Input: part model. Units: mm. Frame: model coordinates. Coordinates: 2 decimals unless noted, no trailing zeros. Loops run counter-clockwise (first coordinate to the right, second up) from the corner with the lowest first, then second, coordinate; pieces in that order, holes last.
```python
from build123d import *

# Parameters (mm, degrees)
SKETCH1_W                    = 139.7
SKETCH1_H                    = 457.2
SKETCH1_R                    = 50.8
SKETCH1_R_2                  = 5.08
BOSS_EXTRUDE1_DEPTH          = 9.652
SKETCH4_W                    = 10.16
SKETCH4_H                    = 7.62
CUT_EXTRUDE1_DEPTH           = 10.652
CHAMFER1_SIZE                = 25.4
SKETCH5_W                    = 76.2
SKETCH5_H                    = 9.652
BOSS_EXTRUDE2_DEPTH          = 4.318
F_3_0_3_DIAMETER_HOLE1_D     = 3
F_3_0_3_DIAMETER_HOLE1_DEPTH = 9.652
SKETCH10_R                   = 1.167867484
SKETCH10_R_2                 = 1.416247351
CUT_EXTRUDE2_DEPTH           = 9.652


with BuildPart() as part:
    # Sketch1 → Boss-Extrude1 (new body)
    with BuildSketch(Plane(origin=(0, 0, 0), x_dir=(1, 0, 0), z_dir=(0, 1, 0))):
        with Locations((69.85, 228.6)):
            Rectangle(SKETCH1_W, SKETCH1_H)
        with Locations((69.85, 228.6)):
            Circle(SKETCH1_R, mode=Mode.SUBTRACT)
        with Locations((38.1, 127)):
            Circle(SKETCH1_R_2, mode=Mode.SUBTRACT)
        with Locations((38.1, 330.2)):
            Circle(SKETCH1_R_2, mode=Mode.SUBTRACT)
    extrude(amount=BOSS_EXTRUDE1_DEPTH)

    # Sketch4 → Cut-Extrude1 (cut, through all)
    with BuildSketch(Plane(origin=(0, 9.652, 0), x_dir=(1, 0, 0), z_dir=(0, 1, 0))):
        with Locations((5.08, 453.39)):
            Rectangle(SKETCH4_W, SKETCH4_H)
    extrude(amount=-CUT_EXTRUDE1_DEPTH, mode=Mode.SUBTRACT)

    # Chamfer1
    chamfer1_edges = [part.edges().sort_by_distance(p)[0] for p in [
        (139.7, 4.826, -457.2),
        (139.7, 4.826, 0),
    ]]
    chamfer(chamfer1_edges, length=CHAMFER1_SIZE)

    # Sketch5 → Boss-Extrude2 (add)
    with BuildSketch(Plane(origin=(139.7, 0, 0), x_dir=(0, 0, -1), z_dir=(1, 0, 0))):
        with Locations((69.85, 4.826)):
            Rectangle(SKETCH5_W, SKETCH5_H)
        with Locations((228.6, 4.826)):
            Rectangle(SKETCH5_W, SKETCH5_H)
        with Locations((387.35, 4.826)):
            Rectangle(SKETCH5_W, SKETCH5_H)
    extrude(amount=BOSS_EXTRUDE2_DEPTH)

    # Ø3.0 (3) Diameter Hole1
    with Locations(Plane(origin=(0, 9.652, 0), x_dir=(1, 0, 0), z_dir=(0, 1, 0))):
        with Locations((109.22, 189.23), (30.48, 189.23), (30.48, 267.97), (109.22, 267.97)):
            Hole(F_3_0_3_DIAMETER_HOLE1_D / 2, depth=F_3_0_3_DIAMETER_HOLE1_DEPTH)

    # Sketch10 → Cut-Extrude2 (cut)
    with BuildSketch(Plane(origin=(0, 9.652, 0), x_dir=(1, 0, 0), z_dir=(0, 1, 0))):
        with Locations((65.024, 49.53)):
            Circle(SKETCH10_R)
        with Locations((69.85, 57.15)):
            Circle(SKETCH10_R_2)
    cut_extrude2 = extrude(amount=-CUT_EXTRUDE2_DEPTH, mode=Mode.SUBTRACT)

    # Mirror1: Cut-Extrude2 across plane
    add(cut_extrude2.mirror(Plane.XY.offset(-228.6)), mode=Mode.SUBTRACT)


solid = part.part
```
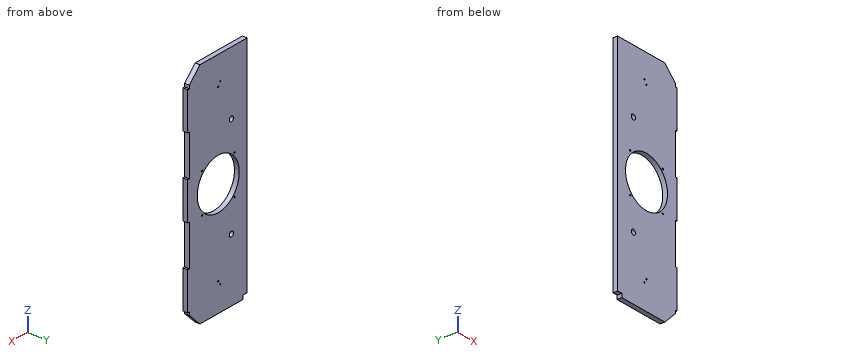
Item 1: Line query: L1, parallel to Z at x = 69.85, y = 4; L2, parallel to X at y = 6.75, z = -400.05; L3, parallel to X at y = 2.5, z = -228.6. Output: solid intervals per line, ascending.
Result:
L1: z = -457.2 to -401.47, -398.63 to -279.4, -177.8 to -58.57, -55.73 to 0
L2: x = 0 to 68.43, 71.27 to 144.02
L3: x = 0 to 19.05, 120.65 to 144.02
Item 2: Section query C-C (x = 91). Output: boundary loops of the cut face in (y, z).
Result:
outline: (0, -457.2) - (9.65, -457.2) - (9.65, -274.79) - (0, -274.79) - close; (0, -182.41) - (9.65, -182.41) - (9.65, 0) - (0, 0) - close
Item 3: Section query D-D (z = -147.5). Output: boundary loops of the cut face in (x, y), then the cut area to 3 significant figures.
Result:
outline: (0, 0) - (139.7, 0) - (139.7, 9.65) - (0, 9.65) - close
area: 1,350 mm2
Item 4: Contact query for flat-ended pins moving along their axis: P1, Ø5, axis at x = 17.5, z = -217.5, coming from the -Y side; P2, Ø1.8, axis at x = 30.48, z = -189.23, coming from the -Y side; P3, Ø4.5, axis at x = 141.5, y = 2.5, coming from the -Z side; P4, Ø1.3, axis at x = 141, y = 5.5, coming from the +Z side. Output: stop coordinate, or through.
Result:
P1: stops at y = 0
P2: passes through
P3: stops at z = -432.25
P4: stops at z = -31.75
Item 5: Section query A-A (z = -228.6). Output: boundary loops of the cut face in (x, y).
Result:
outline: (0, 0) - (19.05, 0) - (19.05, 9.65) - (0, 9.65) - close; (120.65, 0) - (144.02, 0) - (144.02, 9.65) - (120.65, 9.65) - close
Item 6: Section query B-B (y = 5.75). Count the separate pieces of the cut face and the enclosed holes in it, then the cut area to 3 significant figures.
Result:
separate pieces: 1
enclosed holes: 11
area: 55,800 mm2
